```python
from build123d import *

# Parameters (mm, degrees)
BOSS_EXTRUDE1_DEPTH      = 2
BOSS_EXTRUDE2_DEPTH      = 6
SKETCH24_R               = 3.9
BOSS_EXTRUDE5_DEPTH      = 2.3
SKETCH30_W               = 2.408612022
SKETCH30_H               = 1.324178481
CUT_EXTRUDE12_DEPTH      = 8
CUT_EXTRUDE11_DEPTH      = 23.432788503
FILLET1_R                = 1.5
SKETCH34_R               = 0.75
CUT_EXTRUDE13_DEPTH      = 8
SKETCH35_R               = 0.75
CUT_EXTRUDE14_DEPTH      = 3
CUT_EXTRUDE14_DEPTH_BACK = 8
SKETCH36_R               = 0.95
CUT_EXTRUDE15_DEPTH      = 8
SKETCH37_R               = 2
CUT_EXTRUDE16_DEPTH      = 5
SKETCH38_W               = 3
SKETCH38_H               = 1.25
CUT_EXTRUDE17_DEPTH      = 3.6


with BuildPart() as part:
    # Sketch2 → Boss-Extrude1 (new body)
    with BuildSketch(Plane.XY):
        with BuildLine():
            Line((-2.5, 7.5), (-16.7, 7.5))
            Line((-16.7, 7.5), (-20.7, 3.793442666))
            Line((-20.7, 3.793442666), (-20.7, -4.031648778))
            Line((-20.7, -4.031648778), (-15.7, -7.5))
            Line((-15.7, -7.5), (-6.7, -7.5))
            Line((-6.7, -7.5), (-4.2, -5.6))
            ThreePointArc((-4.2, -5.6), (3.130495168, -6.260990337), (7, 0))
            ThreePointArc((7, 0), (4.949747468, 4.949747468), (0, 7))
            Line((0, 7), (0, 7.5))
            Line((0, 7.5), (-2.5, 7.5))
        make_face()
    extrude(amount=BOSS_EXTRUDE1_DEPTH)

    # Sketch4 → Boss-Extrude2 (add)
    with BuildSketch(Plane.XY.offset(2)):
        Polygon((-15.7, -7.5), (-6.7, -7.5), (-6.759079174, -4.5), (-7.7, -4.5), (-7.7, 2), (-5.5, 2), (-5.5, 5.3), (-2.5, 5.3), (-2.5, 7.5), (-16.7, 7.5), (-20.7, 3.793442666), (-20.7, -4.031648778), align=None)
    extrude(amount=BOSS_EXTRUDE2_DEPTH)

    # Sketch24 → Boss-Extrude5 (add)
    with BuildSketch(Plane.XY.offset(2)):
        Circle(SKETCH24_R)
    extrude(amount=BOSS_EXTRUDE5_DEPTH)

    # Sketch30 → Cut-Extrude12 (cut)
    with BuildSketch(Plane(origin=(-5.5, 0, 0), x_dir=(0, 0, -1), z_dir=(1, 0, 0))):
        with Locations((-3.261593395, 4.63791076)):
            Rectangle(SKETCH30_W, SKETCH30_H)
    extrude(amount=-CUT_EXTRUDE12_DEPTH, mode=Mode.SUBTRACT)

    # Sketch28 → Cut-Extrude11 (cut, through all)
    with BuildSketch(Plane.XY.offset(4.3)):
        with BuildLine():
            Line((-1, 1.732050808), (-1, -1.732050808))
            ThreePointArc((-1, -1.732050808), (2, 0), (-1, 1.732050808))
        make_face()
    extrude(amount=-CUT_EXTRUDE11_DEPTH, mode=Mode.SUBTRACT)

    # Fillet1
    fillet1_edges = [part.edges().sort_by_distance(p)[0] for p in [
        (-11.2, -7.5, 0),
        (-8.35, 7.5, 0),
        (-18.7, 5.646721333, 0),
        (-18.2, -5.765824389, 0),
        (-20.7, -0.119103056, 0),
        (-15.7, -7.5, 4),
        (-20.7, -4.031648778, 4),
        (-20.7, 3.793442666, 4),
        (-16.7, 7.5, 4),
    ]]
    fillet(fillet1_edges, radius=FILLET1_R)

    # Sketch34 → Cut-Extrude13 (cut, along a direction that is not the sketch's normal)
    with BuildSketch(Plane.XZ.offset(-2)):
        with Locations((-7, 8)):
            Circle(SKETCH34_R)
    extrude(amount=-CUT_EXTRUDE13_DEPTH, dir=(0.6685833876565112, -0.7436371788377336, 0), mode=Mode.SUBTRACT)

    # Sketch35 → Cut-Extrude14 (cut, two sides, along a direction that is not the sketch's normal)
    with BuildSketch(Plane(origin=(0, -4.5, 0), x_dir=(1, 0, 0), z_dir=(0, 1, 0))) as cut_extrude14_sk:
        with Locations((-8.259079174, -8)):
            Circle(SKETCH35_R)
    extrude(amount=CUT_EXTRUDE14_DEPTH, dir=(0.5999194182208608, 0.8000604299935998, 0), mode=Mode.SUBTRACT)
    extrude(cut_extrude14_sk.sketch, amount=-CUT_EXTRUDE14_DEPTH_BACK, dir=(0.5999194182208608, 0.8000604299935998, 0), mode=Mode.SUBTRACT)

    # Sketch36 → Cut-Extrude15 (cut)
    with BuildSketch(Plane.XY.offset(8)):
        with Locations((-11.7, 0)):
            Circle(SKETCH36_R)
        with Locations((-16.7, 0)):
            Circle(SKETCH36_R)
    extrude(amount=-CUT_EXTRUDE15_DEPTH, mode=Mode.SUBTRACT)

    # Sketch37 → Cut-Extrude16 (cut)
    with BuildSketch(Plane(origin=(0, 0, 0), x_dir=(-1, 0, 0), z_dir=(0, 0, -1))):
        with Locations((11.7, 0)):
            Circle(SKETCH37_R)
        with Locations((16.7, 0)):
            Circle(SKETCH37_R)
    extrude(amount=-CUT_EXTRUDE16_DEPTH, mode=Mode.SUBTRACT)

    # Sketch38 → Cut-Extrude17 (cut)
    with BuildSketch(Plane.XY.offset(8)):
        with Locations((-4, 5.925)):
            Rectangle(SKETCH38_W, SKETCH38_H)
    extrude(amount=-CUT_EXTRUDE17_DEPTH, mode=Mode.SUBTRACT)


with BuildPart() as body_2:
    # Split2: the piece on the far side of the plane
    add(part.part)
    split(bisect_by=Plane.XY.offset(4.4), keep=Keep.BOTTOM)


with BuildPart() as part_1:
    add(part.part)

    # Split2
    split(bisect_by=Plane.XY.offset(4.4), keep=Keep.TOP)


with BuildPart() as body_3:
    # Mirror2: read off the stored shape, not the designer's step
    # Mirror2: mirrored copy
    add(part_1.part.mirror(Plane.XY.offset(8)))


solid = body_3.part
```
Geometry check sheet. Reference: the model listing, model coordinates, mm. A direction names the side the tool comes from. Coordinates: 2 decimals unless noted, no trailing zeros. Loops run counter-clockwise (first coordinate to the right, second up) from the corner with the lowest first, then second, coordinate; pieces in that order, holes last. Notation, with made-up numbers: (13, 86) - (64, 86) arc R4 ccw to (64, 93) - close; hole circle Ø11 at (23, 9). An arc over 180 degrees is marked (long way). One line per item, written item: value. Start each with the question number.
(1) Cross-section at D-D on x = -19.25. Enter the section's corners in (y, z).
(2) Mould release check, pull along Y, two halves, no side actions. Record for faces 4 (the flat face through (-18.098, -5.837, 9.825)), 5 (the flat face through (-8, -6, 8)), 6 (the flat face through (-7.7, -1, 10)), 7 (the flat face through (-9, 5, 11.534)): released by +Y, released by -Y, zero draft, split by the parting line, or undercut.
(3) Cross-section at C-C on x = -16.7. Enter the section's corners in (y, z).
(4) Cross-section at B-B on z = 9.35. Enter the section's corners in (x, y), plus the area to 3 significant figures.
(5) Tool access check on faces 1 (the cylindrical face through (-12.623, -1.774, 11.304)), 2 (the flat face through (-7, 2, 10)), 3 (the flat face through (-5.5, 4, 10)). Record the directions out of +Z, -Z, +X, -X, +Y, -Y that give a thin tool (end or side, any length) a straight path to the whole face; none if there is none.
(6) Material ranges on line 1 (Y direction, x = -11.7, z = 9.5); line 2 (X direction, y = 0.5, z = 11.4); line 3 (X direction, y = 2.5, z = 9.05), recorded low to high. Write a range as [from, to].
(7) Depth check by flat-ended pin: P1, Ø1.8, axis at y = 3, z = 10, coming from the +X side. Enter the tip coordinate at first touch or a pass-through.
(8) Cross-section at A-A on y = 0. Enter the section's corners in (x, z), plus the area to 3 significant figures.
Results below:
1. outline: (-5.04, 8) - (5.14, 8) - (5.14, 11.6) - (-5.04, 11.6) - close
2. face 4: released by -Y
2. face 5: zero draft
2. face 6: undercut
2. face 7: undercut
3. outline: (-6.81, 8) - (-0.95, 8) - (-0.95, 11) - (-2, 11) - (-2, 11.6) - (-6.81, 11.6) - close; (0.95, 8) - (7.38, 8) - (7.38, 11.6) - (2, 11.6) - (2, 11) - (0.95, 11) - close
4. outline: (-20.7, -3.25) arc R1.5 ccw to (-20.05, -4.48) - (-16.09, -7.23) arc R1.5 ccw to (-15.23, -7.5) - (-6.7, -7.5) - (-6.76, -4.5) - (-7.7, -4.5) - (-7.7, 2) - (-5.5, 2) - (-5.5, 6.55) - (-2.5, 6.55) - (-2.5, 7.5) - (-16.11, 7.5) arc R1.5 ccw to (-17.13, 7.1) - (-20.22, 4.24) arc R1.5 ccw to (-20.7, 3.14) - close; hole circle Ø1.9 at (-16.7, 0); hole circle Ø1.9 at (-11.7, 0)
4. area: 191 mm2
5. face 1: +Z
5. face 2: +Z, -Z, +X
5. face 3: +Z, -Z, +X, -Y
6. line 1: y = [-7.5, -0.95], [0.95, 7.5]
6. line 2: x = [-20.7, -18.64], [-14.76, -13.64], [-9.76, -7.7]
6. line 3: x = [-20.7, -5.5]
7. P1: stops at x = -5.5
8. outline: (-20.7, 8) - (-17.65, 8) - (-17.65, 11) - (-18.7, 11) - (-18.7, 11.6) - (-20.7, 11.6) - close; (-15.75, 8) - (-12.65, 8) - (-12.65, 11) - (-13.7, 11) - (-13.7, 11.6) - (-14.7, 11.6) - (-14.7, 11) - (-15.75, 11) - close; (-10.75, 8) - (-7.7, 8) - (-7.7, 11.6) - (-9.7, 11.6) - (-9.7, 11) - (-10.75, 11) - close
8. area: 30.6 mm2
